For this review, use the dimensioned drawing (mm, ordinates from the lowest corner) and the shaded views. A direction names the side the tool comes from. Round coordinates to 2 decimals unless told otherwise and drop trailing zeros. Loops run counter-clockwise (first coordinate to the right, second up) from the corner with the lowest first, then second, coordinate; pieces in that order, holes last. Notation, with made-up numbers: (30, -14.5) - (60, -14.5) arc R17 ccw to (60, -3.5) - close; hole circle Ø5 at (-27, 70). An arc over 180 degrees is marked (long way). Use one line per item in the form item = value. Start each with the question number.
(1) Machinability: for the marked faces 1, 2 and 3, which of the approach directions +Z, -Z, +X, -X, +Y, -Y give a long, thin tool a straight path to every point of the face, cutting with its end or side? Answer none if there is none.
(2) For pin 1 (4 mm diameter, centred on x = 116, z = 84, fed in from +Y); pin 2 (2.5 mm diameter, centred on x = 185, z = 148, fed in from -Y); pin 3 (1.5 mm diameter, centred on x = 113.5, y = 25, fed in from +Z); pin 4 (5 mm diameter, centred on y = 15.5, z = 8.5, fed in from +X), all flat-tipped, find the tip position at first contact; note any pin that passes through.
(3) We need section B-B, the plane z = 135. Write out the cut boundary in (x, y).
(4) We need section A-A, the plane y = 26.5. Write out the cut boundary in (x, z).
(5) We need section C-C, the plane y = 13. Write out the cut boundary in (x, z).
(6) Wall thickness on probe 1 along X at (y, z) = (1, 73); probe 2 along Z at (x, y) = (55, 2.55); probe 3 along X at (y, z) = (2.5, 90.5): over which ranges is each line inside the solid? List them lowest first. Write a range as [from, to].
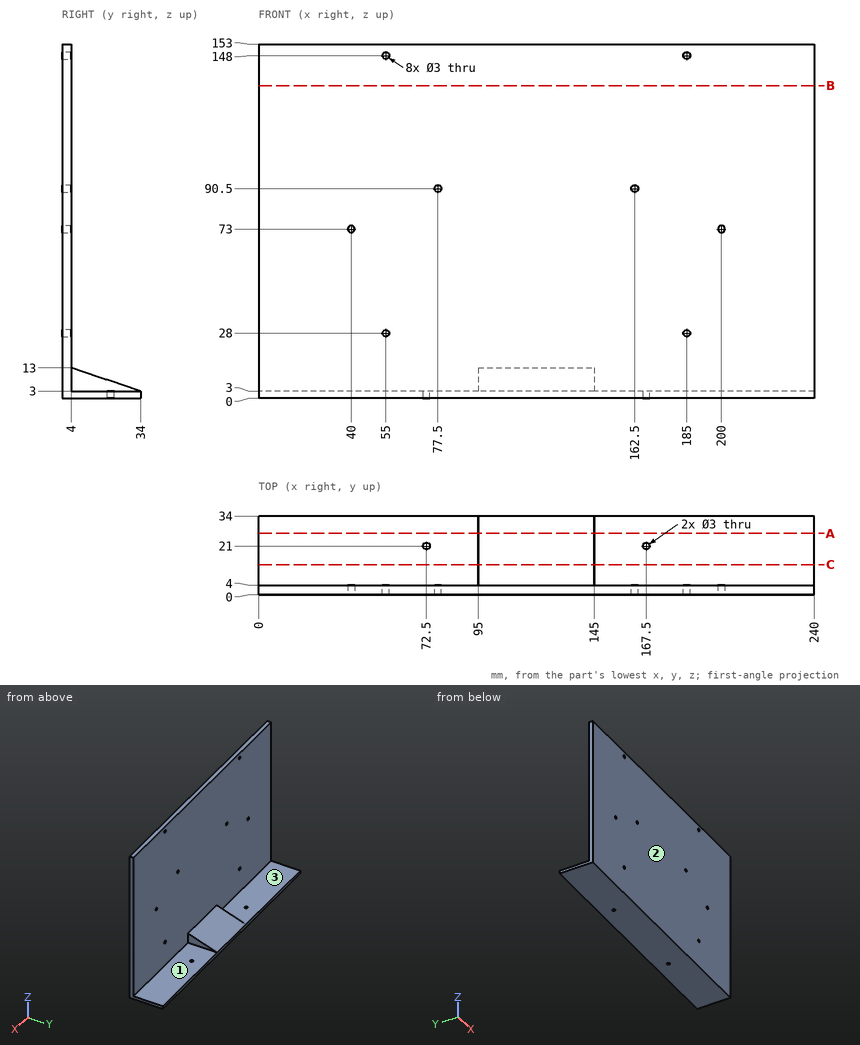
Data:
q1.face_1 = +Z, +X, +Y
q1.face_2 = +Z, -Z, +X, -X, -Y
q1.face_3 = +Z, -X, +Y
q2.pin_1 = 4
q2.pin_2 = through
q2.pin_3 = 6.25
q2.pin_4 = 145
q3.outline = (0, 0) - (240, 0) - (240, 4) - (0, 4) - close
q4.outline = (0, 0) - (240, 0) - (240, 3) - (145, 3) - (145, 5.5) - (95, 5.5) - (95, 3) - (0, 3) - close
q5.outline = (0, 0) - (240, 0) - (240, 3) - (145, 3) - (145, 10) - (95, 10) - (95, 3) - (0, 3) - close
q6.probe_1 = [0, 38.5], [41.5, 198.5], [201.5, 240]
q6.probe_2 = [0, 26.5], [29.5, 146.5], [149.5, 153]
q6.probe_3 = [0, 76], [79, 161], [164, 240]
